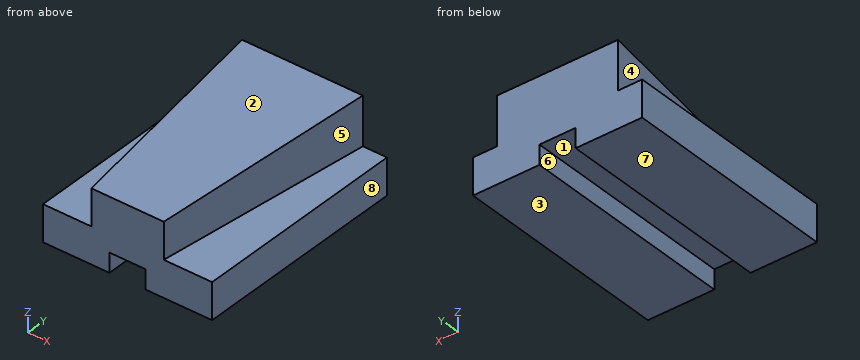
Solid Edge part; units mm, degrees
sketch "Sketch1" plane through (0, 0, 0) normal (0, -1, 0) x (1, 0, 0)
  line L0 (70, 15) -> (0, 15)
  line L1 (0, 15) -> (0, 0)
  line L2 (0, 0) -> (27.5, 0)
  line L3 (27.5, 0) -> (27.5, 8)
  line L4 (27.5, 8) -> (42.5, 8)
  line L5 (42.5, 8) -> (42.5, 0)
  line L6 (42.5, 0) -> (70, 0)
  line L7 (70, 0) -> (70, 15)
extrude "Protrusion1" add sketch "Sketch1" against normal blind 90
sketch "Sketch2" plane through (35, 45, 15) normal (0, 0, 1) x (1, 0, 0)
  line L0 (25, 45) -> (15, -45)
  line L1 (15, -45) -> (-15, -45)
  line L2 (-15, -45) -> (-25, 45)
  line L3 (-25, 45) -> (25, 45)
extrude "ExtrudedProtrusion_3" add sketch "Sketch2" along normal blind 20
extrude "Protrusion2" [suppressed]
sketch "Sketch3" plane through (70, 45, 17.5) normal (1, 0, 0) x (0, 1, 0)
  line L0 (-45, 17.5) -> (-45, 12.5)
  line L1 (-45, 12.5) -> (45, 17.5)
  line L2 (45, 17.5) -> (-45, 17.5)
extrude "ExtrudedCutout_2" cut sketch "Sketch3" against normal blind 76 and the other way blind 76
Source: CAD feature listing. Evaluate the final solid. Frame: model axes, mm. Face numbers are marked on the shaded views. A direction names the side the tool comes from. Round coordinates to 2 decimals unless told otherwise and drop trailing zeros. Write each loop counter-clockwise with the first axis right and the second up, starting at its lowest first coordinate (ties: lowest second). Pieces come first, ordered by that corner, then holes. Notation, with made-up numbers: M 63,3.25 L 108,3.25 A11 cw 108,20.25 Z; hole C 27,88 d10. An arc over 180 degrees is marked long. Answer as a JSON object with one key per item and string values. Group by question number.
(1) Section query B-B on y = 27. Output: boundary loops of the cut face in (x, z).
(2) Mould query, pull axis X, two halves, no side actions, for the marked faces 6, 7 and 8. Classes: +X half, -X half, draft (parallel to the pull), parting line (faces both ways), or undercut.
(3) First-contact query: pin 1 (10 mm diameter, centred on x = 44, z = 21, fed in from -Y); pin 2 (1.5 mm diameter, centred on x = 37.5, y = 58.5, fed in from +Z); pin 3 (6 mm diameter, centred on x = 18, y = 46, fed in from +Z); pin 4 (16 mm diameter, centred on x = 64, y = 37, fed in from +Z). Flat tips, straight axial feed; report the tip coordinate or a pass-through.
(4) Reachability of the marked faces 1, 2, 3, 4 and 5 from +Z, -Z, +X, -X, +Y, -Y: full face, straight path, thin tool, end or side. Return the list, or none.
(5) Section query D-D on z = 17. Output: boundary loops of the cut face in (x, y), then the cut area to 3 significant figures.
(6) Section query A-A on z = 6. Output: boundary loops of the cut face in (x, y).
(7) Ray query, line 1 (X direction, y = 20.5, z = 4); line 2 (Z direction, x = 67, y = 34); line 3 (Z direction, x = 47, y = 32). Return the intervals inside material, ascending. Write a range as [from, to].
(8) Section query C-C on x = 51.5. Output: boundary loops of the cut face in (y, z), then the cut area to 3 significant figures.
Computed values:
{
 "1": {"outline": "M 0,0 L 27.5,0 L 27.5,8 L 42.5,8 L 42.5,0 L 70,0 L 70,15 L 53,15 L 53,31.5 L 17,31.5 L 17,15 L 0,15 Z"},
 "2": {"face 6": "undercut", "face 7": "draft", "face 8": "+X half"},
 "3": {"pin 1": "y = 0", "pin 2": "z = 33.29", "pin 3": "z = 32.72", "pin 4": "z = 15"},
 "4": {"face 1": "-Z, +Y, -Y", "face 2": "+Z, +X, -X, -Y", "face 3": "-Z, +X, -X, +Y, -Y", "face 4": "+Z, -X, -Y", "face 5": "+Z, +X, -Y"},
 "5": {"outline": "M 10,90 L 20,0 L 50,0 L 60,90 Z", "area": "3,600 mm^2"},
 "6": {"outline": "M 0,0 L 27.5,0 L 27.5,90 L 0,90 Z; M 42.5,0 L 70,0 L 70,90 L 42.5,90 Z"},
 "7": {"line 1": "[0, 27.5], [42.5, 70]", "line 2": "[0, 15]", "line 3": "[0, 31.78]"},
 "8": {"outline": "M 0,0 L 90,0 L 90,35 L 13.5,30.75 L 13.5,15 L 0,15 Z", "area": "2,720 mm^2"}
}
